Autodesk Inventor part; units mm, degrees
ref_plane "YZ Plane" through (0, 0, 0) normal (1, 0, 0) x (0, 1, 0)
ref_plane "XZ Plane" through (0, 0, 0) normal (0, 1, 0) x (-1, 0, 0)
ref_plane "XY Plane" through (0, 0, 0) normal (0, 0, 1) x (1, 0, 0)
sketch "Sketch1" plane through (0, 0, 0) normal (0, 0, 1) x (1, 0, 0)
  line L0 (0, 0) -> (24.7, 0) construction
  line L1 (0, 59) -> (3, 59)
  line L2 (3, 92.5) -> (19, 92.5)
  line L3 (3, 92.5) -> (3, 59)
  line L4 (19, 92.5) -> (19, 52)
  line L5 (24.7, 38.5) -> (24.7, 0) construction
  line L6 (19, 52) -> (24.7, 52)
  line L7 (24.7, 52) -> (24.7, 38.5)
  line L8 (24.7, 38.5) -> (12.35, 38.5)
  line L9 (12.35, 38.5) -> (12.35, 32.5)
  line L10 (12.35, 32.5) -> (0, 32.5)
  line L11 (0, 32.5) -> (0, 0) construction
  line L12 (0, 59) -> (0, 32.5)
  dimension "d0" = 118
  dimension "d1" = 185
  dimension "d2" = 104
  dimension "d7" = 77
  dimension "d8" = 65
  dimension "d9" = 19
  dimension "d10" = 3
  dimension "d12" = 12.35
  dimension "d13" = 24.7
revolve "Revolution1" add sketch "Sketch1" angle 360 about axis through (0, 0, 0) along (1, 0, 0)
sketch "Sketch2" plane through (3, 0, 0) normal (-1, 0, 0) x (0, 0, 1)
  circle A0 centre (0, 0) radius 59
  line L0 (0, 0) -> (0, 72.5) construction
  circle A1 centre (0, 0) radius 92.5
  circle A2 centre (0, 0) radius 72.5 construction
  line L1 (0, 0) -> (27.7445, 66.9813) construction
  circle A3 centre (27.7445, 66.9813) radius 9.5
  dimension "d14" = 19
  dimension "d15" = 72.5
  dimension "d16" = 22.5
extrude "Extrusion1" cut sketch "Sketch2" against normal blind 19 contours A3
pattern_circular "Circular Pattern1" count 8 over 360 about axis through (1.5, 0, 0) along (1, 0, 0) of "Extrusion1"
equation "\"d0\" = D1"
equation "\"d1\" = D"
equation "\"d2\" = N3"
equation "\"d7\" = ID + 2 * t"
equation "\"d8\" = ID"
equation "\"d9\" = C1"
equation "\"d10\" = F1"
equation "\"d12\" = 0.65 * C1"
equation "\"d13\" = 1.3 * C1"
equation "\"d14\" = L"
equation "\"d15\" = 0.5 * K1"
equation "\"d3\" = C1"
equation "\"C1\" = 19"
equation "\"D\" = 185"
equation "\"K1\" = 145"
equation "\"L\" = 19"
equation "\"N3\" = 104"
equation "\"D1\" = 118"
equation "\"H1\" = 17"
equation "\"F1\" = 3"
equation "\"ID\" = 65"
equation "\"t\" = 6"
equation "\"Size_Designation\" = 1.2345"
properties part number "DIN EN 1092-2 Hubbed Socket Welding Flange Type 14 - PN 40 Ductile Iron DN65" material "Iron, Ductile"
Part model, mm, in its own coordinate system. A direction names the side the tool comes from. Coordinates: 2 decimals unless noted, no trailing zeros. Write each loop counter-clockwise with the first axis right and the second up, starting at its lowest first coordinate (ties: lowest second). Pieces come first, ordered by that corner, then holes.
Item 1: Slice it at C-C (z = 62). Write the cut outline in (x, y).
Item 2: Which spindle directions (+Z, -Z, +X, -X, +Y, -Y) get a long thin tool onto all of the face, cutting with end or side? Do faces 4 (the face through (0, 25, -25)), 5 (the face through (18.44, -30.55, 23.43)), 6 (the face through (3, -1, -60)). Say none if no direction does.
Item 3: Slice it at D-D (x = 10). Count the separate pieces of the cut face and the enclosed holes in it, and give its area (3 significant figures).
Item 4: Mould opens along Y. For faces 1 (the face through (10.888, -57.707, -25.685)), 2 (the face through (19, 40, -40)), 3 (the face through (11.112, 49.727, 77.996)) say: released by +Y, released by -Y, zero draft, split by the parting line, or undercut.
Item 5: Slice it at A-A (y = 0). Write the cut outline in (x, z).
Item 6: Pin check, flat tips, straight feed: pin 1 (24.5 mm diameter, centred on y = -66.98, z = 27.74, fed in from -X); pin 2 (3 mm diameter, centred on x = 3.5, z = 67.5, fed in from +Y); pin 3 (15 mm diameter, centred on y = 66.98, z = -27.74, fed in from -X); pin 4 (4 mm diameter, centred on x = 9, y = 21, fed in from -Z). Stop position of each tip, or through.
Item 7: Probe line 1 (Z direction, x = 8.5, y = 72.5); line 2 (Z direction, x = 4, y = 23.5); line 3 (Z direction, x = 15, y = -26.5). List the from-to ranges inside material, lowest first.
Results found:
1. outline: (3, -68.65) - (19, -68.65) - (19, -35.83) - (3, -35.83) - close; (3, -19.66) - (19, -19.66) - (19, 19.66) - (3, 19.66) - close; (3, 35.83) - (19, 35.83) - (19, 68.65) - (3, 68.65) - close
2. face 4: +Z, -Z, -X, +Y, -Y
2. face 5: +X
2. face 6: -X
3. separate pieces: 1
3. enclosed holes: 9
3. area: 21,300 mm2
4. face 1: undercut
4. face 2: zero draft
4. face 3: split by the parting line
5. outline: (0, -59) - (3, -59) - (3, -92.5) - (19, -92.5) - (19, -52) - (24.7, -52) - (24.7, -38.5) - (12.35, -38.5) - (12.35, -32.5) - (0, -32.5) - close; (0, 32.5) - (12.35, 32.5) - (12.35, 38.5) - (24.7, 38.5) - (24.7, 52) - (19, 52) - (19, 92.5) - (3, 92.5) - (3, 59) - (0, 59) - close
6. pin 1: stops at x = 3
6. pin 2: stops at y = 64.81
6. pin 3: passes through
6. pin 4: stops at z = -90.53
7. line 1: z = -57.45 to -35.48, -20.01 to 20.01, 35.48 to 57.45
7. line 2: z = -89.47 to -75.48, -58.48 to -22.45, 22.45 to 58.48, 75.48 to 89.47
7. line 3: z = -88.62 to -76.4, -57.56 to -27.93, 27.93 to 57.56, 76.4 to 88.62
